from build123d import *

# Parameters (mm, degrees)
SKETCH1_R           = 1.7
BOSS_EXTRUDE2_DEPTH = 3
SKETCH1_5_R         = 3.15
SKETCH1_5_R_2       = 1.7
SKETCH1_5_W         = 25
SKETCH1_5_H         = 3
BOSS_EXTRUDE3_DEPTH = 3.6
BOSS_EXTRUDE4_START = 3.6
SKETCH1_7_W         = 25
SKETCH1_7_H         = 3
BOSS_EXTRUDE4_DEPTH = 16
CUT_EXTRUDE1_REACH  = 26
SKETCH2_R           = 1.1
SKETCH2_R_2         = 6.5
CUT_EXTRUDE2_REACH  = 5


with BuildPart() as part:
    # Sketch1 → Boss-Extrude2 (new body)
    with BuildSketch(Plane(origin=(0, 0, 0), x_dir=(1, 0, 0), z_dir=(0, 1, 0))):
        with BuildLine():
            ThreePointArc((24.595917942, -46), (19.595917942, -41), (14.595917942, -46))
            Line((14.595917942, -46), (14.595917942, -53.027909439))
            ThreePointArc((14.595917942, -53.027909439), (0, -55), (-14.595917942, -53.027909439))
            Line((-14.595917942, -53.027909439), (-14.595917942, -46))
            ThreePointArc((-14.595917942, -46), (-19.595917942, -41), (-24.595917942, -46))
            Line((-24.595917942, -46), (-24.595917942, -61.451532288))
            ThreePointArc((-24.595917942, -61.451532288), (-18.632624286, -63.514370911), (-12.5, -65))
            Line((-12.5, -65), (12.5, -65))
            ThreePointArc((12.5, -65), (18.632624286, -63.514370911), (24.595917942, -61.451532288))
            Line((24.595917942, -61.451532288), (24.595917942, -46))
        make_face()
        with Locations((-19.595917942, -46)):
            Circle(SKETCH1_R, mode=Mode.SUBTRACT)
        with Locations((19.595917942, -46)):
            Circle(SKETCH1_R, mode=Mode.SUBTRACT)
    extrude(amount=-BOSS_EXTRUDE2_DEPTH)

    # Sketch1<5> → Boss-Extrude3 (add)
    with BuildSketch(Plane(origin=(0, 0, 0), x_dir=(1, 0, 0), z_dir=(0, 1, 0))):
        with Locations((-19.595917942, -46)):
            Circle(SKETCH1_5_R)
        with Locations((-19.595917942, -46)):
            Circle(SKETCH1_5_R_2, mode=Mode.SUBTRACT)
        with Locations((19.595917942, -46)):
            Circle(SKETCH1_5_R)
        with Locations((19.595917942, -46)):
            Circle(SKETCH1_5_R_2, mode=Mode.SUBTRACT)
        with Locations((0, -63.5)):
            Rectangle(SKETCH1_5_W, SKETCH1_5_H)
    extrude(amount=BOSS_EXTRUDE3_DEPTH)

    # Sketch1<7> → Boss-Extrude4 (add)
    with BuildSketch(Plane(origin=(0, 0, 0), x_dir=(1, 0, 0), z_dir=(0, 1, 0)).offset(BOSS_EXTRUDE4_START)):
        with Locations((0, -63.5)):
            Rectangle(SKETCH1_7_W, SKETCH1_7_H)
    extrude(amount=BOSS_EXTRUDE4_DEPTH)

    # Sketch2 → Cut-Extrude1 (cut, up to next)
    with BuildSketch(Plane.XY.offset(65), mode=Mode.PRIVATE) as cut_extrude1_sk1:
        with Locations((-10.5, 4)):
            Circle(SKETCH2_R)
    cut_extrude1_tool1 = extrude(cut_extrude1_sk1.sketch, amount=-CUT_EXTRUDE1_REACH, mode=Mode.PRIVATE) & part.part
    add(cut_extrude1_tool1.solids().sort_by_distance((-10.5, 4, 65))[0], mode=Mode.SUBTRACT)
    # Sketch2 → Cut-Extrude1 (cut, up to next)
    with BuildSketch(Plane.XY.offset(65), mode=Mode.PRIVATE) as cut_extrude1_sk2:
        with Locations((-10.5, 16.5)):
            Circle(SKETCH2_R)
    cut_extrude1_tool2 = extrude(cut_extrude1_sk2.sketch, amount=-CUT_EXTRUDE1_REACH, mode=Mode.PRIVATE) & part.part
    add(cut_extrude1_tool2.solids().sort_by_distance((-10.5, 16.5, 65))[0], mode=Mode.SUBTRACT)
    # Sketch2 → Cut-Extrude1 (cut, up to next)
    with BuildSketch(Plane.XY.offset(65), mode=Mode.PRIVATE) as cut_extrude1_sk3:
        with Locations((10.5, 4)):
            Circle(SKETCH2_R)
    cut_extrude1_tool3 = extrude(cut_extrude1_sk3.sketch, amount=-CUT_EXTRUDE1_REACH, mode=Mode.PRIVATE) & part.part
    add(cut_extrude1_tool3.solids().sort_by_distance((10.5, 4, 65))[0], mode=Mode.SUBTRACT)
    # Sketch2 → Cut-Extrude1 (cut, up to next)
    with BuildSketch(Plane.XY.offset(65), mode=Mode.PRIVATE) as cut_extrude1_sk4:
        with Locations((10.5, 16.5)):
            Circle(SKETCH2_R)
    cut_extrude1_tool4 = extrude(cut_extrude1_sk4.sketch, amount=-CUT_EXTRUDE1_REACH, mode=Mode.PRIVATE) & part.part
    add(cut_extrude1_tool4.solids().sort_by_distance((10.5, 16.5, 65))[0], mode=Mode.SUBTRACT)
    # Sketch2 → Cut-Extrude1 (cut, up to next)
    with BuildSketch(Plane.XY.offset(65), mode=Mode.PRIVATE) as cut_extrude1_sk5:
        with Locations((0, 10.25)):
            Circle(SKETCH2_R_2)
    cut_extrude1_tool5 = extrude(cut_extrude1_sk5.sketch, amount=-CUT_EXTRUDE1_REACH, mode=Mode.PRIVATE) & part.part
    add(cut_extrude1_tool5.solids().sort_by_distance((0, 10.25, 65))[0], mode=Mode.SUBTRACT)

    # Sketch3 → Cut-Extrude2 (cut, up to next)
    with BuildSketch(Plane(origin=(0, 0, 0), x_dir=(1, 0, 0), z_dir=(0, 1, 0)), mode=Mode.PRIVATE) as cut_extrude2_sk1:
        with BuildLine():
            Line((-15.5, -61.260541388), (-15.5, -59))
            Line((-15.5, -59), (15.5, -59))
            Line((15.5, -59), (15.5, -61.260541388))
            ThreePointArc((15.5, -61.260541388), (18.571620144, -60.400321658), (21.595917942, -59.386195866))
            Line((21.595917942, -59.386195866), (21.595917942, -50.745787606))
            ThreePointArc((21.595917942, -50.745787606), (19.595917942, -51.15), (17.595917942, -50.745787606))
            Line((17.595917942, -50.745787606), (17.595917942, -55.266478735))
            ThreePointArc((17.595917942, -55.266478735), (0, -58), (-17.595917942, -55.266478735))
            Line((-17.595917942, -55.266478735), (-17.595917942, -50.745787606))
            ThreePointArc((-17.595917942, -50.745787606), (-19.595917942, -51.15), (-21.595917942, -50.745787606))
            Line((-21.595917942, -50.745787606), (-21.595917942, -59.386195866))
            ThreePointArc((-21.595917942, -59.386195866), (-18.571620144, -60.400321658), (-15.5, -61.260541388))
        make_face()
    cut_extrude2_tool1 = extrude(cut_extrude2_sk1.sketch, amount=-CUT_EXTRUDE2_REACH, mode=Mode.PRIVATE) & part.part
    add(cut_extrude2_tool1.solids().sort_by_distance((-18.040451, 0, 53.006133))[0], mode=Mode.SUBTRACT)


solid = part.part
Could you check a few things on this model? Use its own coordinates, in mm. A direction names the side the tool comes from. Coordinates: 2 decimals unless noted, no trailing zeros. Loops run counter-clockwise (first coordinate to the right, second up) from the corner with the lowest first, then second, coordinate; pieces in that order, holes last. Notation, with made-up numbers: (67.25, 10) -> (93.25, 10) arc R12 ccw to (93.25, 30) -> close; hole circle Ø6 at (60, 12). An arc over 180 degrees is marked (long way). Answer in a Markdown table with one row per item.
(1) Imagine slicing it at A-A (y = 10.25). List the corners of the cut face in (x, z) for me, plus the area to 3 significant figures.
Results found:
| item | result |
|---|---|
| outline | (-12.5, 62) -> (-6.5, 62) -> (-6.5, 65) -> (-12.5, 65) -> close; (6.5, 62) -> (12.5, 62) -> (12.5, 65) -> (6.5, 65) -> close |
| area | 36.0 mm^2 |
(2) Thinking about a two-plate mould opening in Z: for faces 4 (the face through (-0.3, -3, 55.5)), 5 (the face through (0, 3, 65)), 6 (the face through (18.529, -1.479, 60.413)), which applies, released by +Z, released by -Z, zero draft, split by the parting line, or undercut?
Results found:
| item | result |
|---|---|
| face 4 | zero draft |
| face 5 | released by +Z |
| face 6 | undercut |
(3) For faces 1 (the face through (14.596, -1, 49)), 2 (the face through (-12.5, 10, 64)), 3 (the face through (-17.596, -1, 53)), which set-ups out of +Z, -Z, +X, -X, +Y, -Y let a thin tool reach every point of the face, with its end or its side?
Results found:
| item | result |
|---|---|
| face 1 | -Z, +Y, -Y |
| face 2 | +Z, -Z, -X, +Y |
| face 3 | +Y, -Y |
(4) Imagine slicing it at B-B (x = 0). List the corners of the cut face in (y, z) for me.
Results found:
| item | result |
|---|---|
| outline | (-3, 55) -> (0, 55) -> (0, 58) -> (-3, 58) -> close; (-3, 59) -> (0, 59) -> (0, 62) -> (3.75, 62) -> (3.75, 65) -> (-3, 65) -> close; (16.75, 62) -> (19.6, 62) -> (19.6, 65) -> (16.75, 65) -> close |
(5) Will these pins go through, and if not, where does the flat tip stop? pin 1 Ø6 at (x, y) = (-14, 16) entering from -Z; pin 2 Ø3 at (x, z) = (-18, 52.5) entering from -Y; pin 3 Ø7 at (x, z) = (18.5, 45.5) entering from +Y; pin 4 Ø1.5 at (y, z) = (6, 63) entering from -X.
Results found:
| item | result |
|---|---|
| pin 1 | stops at z = 62 |
| pin 2 | stops at y = -3 |
| pin 3 | stops at y = 3.6 |
| pin 4 | stops at x = -12.5 |
(6) If I drill on probe 1 along X at (y, z) = (-1, 46); probe 2 along Y at (x, z) = (10.5, 64.2); probe 3 along X at (y, z) = (1.5, 46), over which ranges is the centre line in solid material (lowest first)?
Results found:
| item | result |
|---|---|
| probe 1 | x = -24.6 to -21.3, -17.9 to -14.6, 14.6 to 17.9, 21.3 to 24.6 |
| probe 2 | y = -3 to 2.9, 5.1 to 15.4, 17.6 to 19.6 |
| probe 3 | x = -22.75 to -21.3, -17.9 to -16.45, 16.45 to 17.9, 21.3 to 22.75 |
(7) Imagine slicing it at D-D (x = -8). List the corners of the cut face in (y, z) for me, plus the area to 3 significant figures.
Results found:
| item | result |
|---|---|
| outline | (-3, 54.42) -> (0, 54.42) -> (0, 57.45) -> (-3, 57.45) -> close; (-3, 59) -> (0, 59) -> (0, 62) -> (19.6, 62) -> (19.6, 65) -> (-3, 65) -> close |
| area | 85.9 mm^2 |
(8) Imagine slicing it at C-C (z = 58.5). List the corners of the cut face in (x, y) for me, plus the area to 3 significant figures.
Results found:
| item | result |
|---|---|
| outline | (-24.6, -3) -> (-21.6, -3) -> (-21.6, 0) -> (-24.6, 0) -> close; (21.6, -3) -> (24.6, -3) -> (24.6, 0) -> (21.6, 0) -> close |
| area | 18.0 mm^2 |
